```python
from build123d import *

# Parameters (mm, degrees)
BASES_R                  = 19
BASE_DEPTH               = 3
WALLS_R                  = 10
WALLS_R_2                = 7.5
WALL_DEPTH               = 5
FASTENINGBODYS_R         = 18
FASTENINGBODY_DEPTH      = 8
CIRPATTERN1_COUNT        = 3
BEARINGACCESSBORES_R     = 7
BEARINGACCESSBORE_DEPTH  = 30.03446232
ADDITIONALDEPTHCUT_START = -1
ADDITIONALDEPTHCUTS_R    = 7.5
ADDITIONALDEPTHCUT_DEPTH = 1
CIRPATTERN2_COUNT        = 3
CIRPATTERN3_COUNT        = 3
CHAMFER1_SIZE            = 0.5
CHAMFER2_SIZE            = 0.2


with BuildPart() as part:
    # BaseS → Base (new body)
    with BuildSketch(Plane(origin=(0, 0, 0), x_dir=(0, 0, -1), z_dir=(1, 0, 0))):
        Circle(BASES_R)
    extrude(amount=BASE_DEPTH)

    # WallS → Wall (add)
    with BuildSketch(Plane(origin=(3, 0, 0), x_dir=(0, 0, -1), z_dir=(1, 0, 0))):
        Circle(WALLS_R)
        Circle(WALLS_R_2, mode=Mode.SUBTRACT)
    extrude(amount=WALL_DEPTH)

    # FasteningBodyS → FasteningBody (add)
    with BuildSketch(Plane.ZY):
        Circle(FASTENINGBODYS_R)
    extrude(amount=FASTENINGBODY_DEPTH)

    # Sketch5 → M2x0.4 Tapped Hole1 (revolve, cut)
    with BuildSketch(Plane(origin=(-4, 18, 0), x_dir=(0, 0, 1), z_dir=(1, 0, 0))):
        Polygon((0, 0), (0, 5.680688495), (0.8, 5.2), (0.8, 0), align=None)
    m2x0_4_tapped_hole1 = revolve(axis=Axis((-4, 24.35, 0), (0, -1, 0)), mode=Mode.SUBTRACT)

    # CirPattern1: M2x0.4 Tapped Hole1 ×3 about axis
    cirpattern1_axis = Axis((-8, 0, 0), (1, 0, 0))
    for i in range(1, CIRPATTERN1_COUNT):
        add(m2x0_4_tapped_hole1.rotate(cirpattern1_axis, i * 360 / CIRPATTERN1_COUNT), mode=Mode.SUBTRACT)

    # BearingAccessBoreS → BearingAccessBore (cut, through all)
    with BuildSketch(Plane(origin=(3, 0, 0), x_dir=(0, 0, -1), z_dir=(1, 0, 0))):
        Circle(BEARINGACCESSBORES_R)
    extrude(amount=-BEARINGACCESSBORE_DEPTH, mode=Mode.SUBTRACT)

    # AdditionalDepthCutS → AdditionalDepthCut (cut)
    with BuildSketch(Plane(origin=(3, 0, 0), x_dir=(0, 0, -1), z_dir=(1, 0, 0)).offset(ADDITIONALDEPTHCUT_START)):
        Circle(ADDITIONALDEPTHCUTS_R)
    extrude(amount=ADDITIONALDEPTHCUT_DEPTH, mode=Mode.SUBTRACT)

    # Sketch11 → M3x0.5 Tapped Hole2 (revolve, cut)
    with BuildSketch(Plane(origin=(3, -15, 0), x_dir=(0, 0, -1), z_dir=(0, 1, 0))):
        Polygon((0, 0), (0, 8.251075774), (1.25, 7.5), (1.25, 0), align=None)
    m3x0_5_tapped_hole2 = revolve(axis=Axis((9.35, -15, 0), (-1, 0, 0)), mode=Mode.SUBTRACT)

    # Sketch8 → M3x0.5 Tapped Hole1 (revolve, cut)
    with BuildSketch(Plane(origin=(3, -11.46812862, 8.030070109), x_dir=(0, 0, -1), z_dir=(0, 1, 0))):
        Polygon((0, 0), (0, 8.251075774), (1.25, 7.5), (1.25, 0), align=None)
    m3x0_5_tapped_hole1 = revolve(axis=Axis((9.35, -11.46812862, 8.030070109), (-1, 0, 0)), mode=Mode.SUBTRACT)

    # CirPattern2: M3x0.5 Tapped Hole1 ×3 about axis
    cirpattern2_axis = Axis((0, 0, 0), (1, 0, 0))
    for i in range(1, CIRPATTERN2_COUNT):
        add(m3x0_5_tapped_hole1.rotate(cirpattern2_axis, i * 360 / CIRPATTERN2_COUNT), mode=Mode.SUBTRACT)

    # CirPattern3: M3x0.5 Tapped Hole2 ×3 about axis
    cirpattern3_axis = Axis((0, 0, 0), (1, 0, 0))
    for i in range(1, CIRPATTERN3_COUNT):
        add(m3x0_5_tapped_hole2.rotate(cirpattern3_axis, i * 360 / CIRPATTERN3_COUNT), mode=Mode.SUBTRACT)

    # Chamfer1
    chamfer1_edges = [part.edges().sort_by_distance(p)[0] for p in [
        (8, 0, 7.5),
    ]]
    chamfer(chamfer1_edges, length=CHAMFER1_SIZE)

    # Chamfer2
    chamfer2_edges = [part.edges().sort_by_distance(p)[0] for p in [
        (3, 0, 19),
    ]]
    chamfer(chamfer2_edges, length=CHAMFER2_SIZE)


solid = part.part
```
For this review, take the finished solid that the model builds, in its own axes (mm). A direction names the side the tool comes from. Round coordinates to 2 decimals unless told otherwise and drop trailing zeros. Write each loop counter-clockwise with the first axis right and the second up, starting at its lowest first coordinate (ties: lowest second). Pieces come first, ordered by that corner, then holes. Notation, with made-up numbers: (17, -26) - (55, -26) arc R10 cw to (55, -18) - close; hole circle Ø11 at (-33.75, 47). An arc over 180 degrees is marked (long way). Answer as CSV lines item,"result". Start each with the question number.
(1) Mouldability with a two-part tool opening along Z and no side actions: class faces 1 (the flat face through (0, -17, -7)), 2 (the flat face through (2, 2, -7)), 3 (the cylindrical face through (1.38, -16.856, -8.767)) as +Z half, -Z half, draft (parallel to the pull), parting line (faces both ways), or undercut.
(2) For line 1 (Y direction, x = 1, z = 0); line 2 (Y direction, x = 4, z = 0); line 3 (X direction, y = -2, z = 11.5), list the stretches that pass through material, from the lowest coordinate up.
(3) Machinability: for faces 4 (the cylindrical face through (-0.7, 8.72, 13.26)), 5 (the cylindrical face through (-3.944, 17.847, -2.343)), 6 (the conical face through (-3.947, -6.09, -10.805)), 7 (the cylindrical face through (-3.22, 15.44, -0.17)), 8 (the flat face through (8, 8.2, 0)), which of the approach directions +Z, -Z, +X, -X, +Y, -Y give a long, thin tool a straight path to every point of the face, cutting with its end or side? Answer none if there is none.
(4) For pin 1 (1.8 mm diameter, centred on x = -4, z = 0, fed in from -Y); pin 2 (8 mm diameter, centred on x = 5.5, y = -2, fed in from -Z); pin 3 (2 mm diameter, centred on y = 12.69, z = 5.92, fed in from +X); pin 4 (3 mm diameter, centred on y = -11.47, z = 8.03, fed in from +X), all flat-tipped, find the tip position at first contact; note any pin that passes through.
(5) Add section A-A, the plane x = 5.25. State the section outline as (y, z) points.
From the geometry:
1,face 1,"draft"
1,face 2,"undercut"
1,face 3,"parting line"
2,line 1,"y = -19 to -16.25, -13.75 to -7, 7 to 19"
2,line 2,"y = -10 to -7.5, 7.5 to 10"
2,line 3,"x = -8 to 3"
3,face 4,"+X"
3,face 5,"-X"
3,face 6,"none"
3,face 7,"+Y"
3,face 8,"+Z, -Z, +X, +Y, -Y"
4,pin 1,"stops at y = -18"
4,pin 2,"stops at z = -19"
4,pin 3,"stops at x = -4.65"
4,pin 4,"stops at x = 3"
5,outline,"circle Ø20 at (0, 0); hole circle Ø15 at (0, 0)"
